```python
from build123d import *

# Parameters (mm, degrees)
SKETCH_1_W          = 35
SKETCH_1_H          = 8
EXTRUDE_1_DEPTH     = 28
SKETCH_2_R          = 1.75
CUT_EXTRUDE_1_DEPTH = 29
CUT_EXTRUDE_2_DEPTH = 29
FILLET_1_R          = 2
EXTRUDE_2_DEPTH     = 28


with BuildPart() as part:
    # Эскиз1 → Бобышка-Вытянуть1 (new body)
    with BuildSketch(Plane.XY):
        Polygon((17.5, 4), (17.5, 74), (-17.5, 4), align=None)
        Rectangle(SKETCH_1_W, SKETCH_1_H)
    extrude(amount=EXTRUDE_1_DEPTH)

    # Эскиз2 → Вырез-Вытянуть1 (cut, through all)
    with BuildSketch(Plane.XY.offset(28)):
        Circle(SKETCH_2_R)
        with Locations((-14, 0)):
            Circle(SKETCH_2_R)
        with Locations((14, 0)):
            Circle(SKETCH_2_R)
    extrude(amount=-CUT_EXTRUDE_1_DEPTH, mode=Mode.SUBTRACT)

    # Эскиз3 → Вырез-Вытянуть2 (cut, through all)
    with BuildSketch(Plane.XY.offset(28)):
        Polygon((-13.027864045, 4), (15.5, 4), (15.5, 61.05572809), align=None)
    extrude(amount=-CUT_EXTRUDE_2_DEPTH, mode=Mode.SUBTRACT)

    # Скругление1
    fillet_1_edges = [part.edges().sort_by_distance(p)[0] for p in [
        (17.5, 74, 14),
    ]]
    fillet(fillet_1_edges, radius=FILLET_1_R)

    # Эскиз5 → Бобышка-Вытянуть2 (add)
    with BuildSketch(Plane.XY.offset(28)):
        Polygon((15.5, 12.539466863), (15.5, 10.539418123), (-9.84663286, 10.362462369), (-8.843105462, 12.369517166), align=None)
        Polygon((15.5, 21.269833716), (15.5, 19.269821531), (-5.429482266, 19.196763559), (-4.427727775, 21.200272541), align=None)
        Polygon((-0.027864045, 30), (-1.027864045, 28), (15.5, 28), (15.5, 30), align=None)
        Polygon((4.356674041, 38.769076173), (3.358410255, 36.7725486), (15.5, 36.730166284), (15.5, 38.730178469), align=None)
        Polygon((8.726072744, 47.507873578), (7.729527032, 45.514782153), (15.5, 45.460533137), (15.5, 47.460581877), align=None)
    extrude(amount=-EXTRUDE_2_DEPTH)


solid = part.part
```
CAD build for the part. Positions are in the model's coordinates, mm. A direction names the side the tool comes from. Give positions to 0.01 mm unless a question says otherwise; leave off trailing zeros. Loops run counter-clockwise (first coordinate to the right, second up) from the corner with the lowest first, then second, coordinate; pieces in that order, holes last. Notation, with made-up numbers: M -15.5,-20.5 L -9.5,-20.5 A25 cw -9.5,-7.5 Z; hole C -19.75,79.25 d2. An arc over 180 degrees is marked long. Use one line per item in the form item = value.
Item 1: Flat gauge pins, fed straight in: pin 1 (7 mm diameter, centred on y = 52.5, z = 15, fed in from -X); pin 2 (2 mm diameter, centred on y = 55.5, z = 17, fed in from -X); pin 3 (3.5 mm diameter, centred on y = 40.5, z = 11, fed in from -X) (3 decimals). Where does each tip first touch, or does it go through?
Determined:
pin_1 = 5
pin_2 = 7.75
pin_3 = -0.125
Item 2: Slice it at C-C (z = 18). Count the separate pieces of the cut face and the enclosed holes in it, plus the area to 3 significant figures.
Determined:
separate_pieces = 1
enclosed_holes = 9
area = 811 mm2
Item 3: Slice it at A-A (x = -14). List the corners of the cut face in (y, z).
Determined:
outline = M -4,0 L -1.75,0 L -1.75,28 L -4,28 Z; M 1.75,0 L 11,0 L 11,28 L 1.75,28 Z
Item 4: Drill centre lines: probe 1 along Y at (x, z) = (-2, 10); probe 2 along Y at (x, z) = (-6.5, 15); probe 3 along Y at (x, z) = (-2.5, 6.5). Where is each one in solid material? Low to high. Write a range as from..to.
Determined:
probe_1 = -4..4, 10.42..12.42, 19.21..21.21, 26.06..35
probe_2 = -4..4, 10.39..12.39, 17.06..26
probe_3 = -4..4, 10.41..12.41, 19.21..21.21, 25.06..34
Item 5: Slice it at D-D (y = 17). List the corners of the cut face in (x, z), plus the area to 3 significant figures.
Determined:
outline = M -11,0 L -6.53,0 L -6.53,28 L -11,28 Z; M 15.5,0 L 17.5,0 L 17.5,28 L 15.5,28 Z
area = 181 mm2
Item 6: Slice it at B-B (y = 0). List the corners of the cut face in (x, z), plus the area to 3 significant figures.
Determined:
outline = M -17.5,0 L -15.75,0 L -15.75,28 L -17.5,28 Z; M -12.25,0 L -1.75,0 L -1.75,28 L -12.25,28 Z; M 1.75,0 L 12.25,0 L 12.25,28 L 1.75,28 Z; M 15.75,0 L 17.5,0 L 17.5,28 L 15.75,28 Z
area = 686 mm2
Item 7: Which spindle directions (+Z, -Z, +X, -X, +Y, -Y) get a long thin tool onto all of the face, cutting with end or side? Do faces 5 (the face through (15.5, 7, 14)), 6 (the face through (-1.7, 35.6, 13.8)). Say none if no direction does.
Determined:
face_5 = +Z, -Z
face_6 = +Z, -Z, -X, +Y
Item 8: Two-plate mould, pull along Y, no slides. Class faces 1 (the face through (15.669, 0.526, 14.196)), 2 (the face through (-4, 24, 28)), 3 (the face through (15.923, 67.483, 14.196)), 4 (the face through (1.617, -0.67, 14.196)): pulls with the +Y half, pulls with the -Y half, needs draft (parallel to the pull), parting line crosses it, or undercut.
Determined:
face_1 = undercut
face_2 = needs draft
face_3 = pulls with the +Y half
face_4 = undercut
